```python
from build123d import *

# Parameters (mm, degrees)
SKETCH3_W           = 39.5
SKETCH3_H           = 50
SKETCH3_W_2         = 33.5
SKETCH3_H_2         = 44
BOSS_EXTRUDE1_DEPTH = 2
SKETCH4_W           = 39.5
SKETCH4_H           = 50
BOSS_EXTRUDE2_DEPTH = 1.5
SKETCH5_W           = 1.5
SKETCH5_H           = 11
CUT_EXTRUDE1_DEPTH  = 3
SKETCH7_W           = 39.5
SKETCH7_H           = 50
SKETCH7_W_2         = 28.5
SKETCH7_H_2         = 30.1
BOSS_EXTRUDE3_DEPTH = 1
SKETCH8_W           = 3
SKETCH8_H           = 6.1
SKETCH8_H_2         = 20.2
CUT_EXTRUDE2_DEPTH  = 4.5


with BuildPart() as part:
    # Sketch3 → Boss-Extrude1 (new body)
    with BuildSketch(Plane(origin=(0, 0, 0), x_dir=(1, 0, 0), z_dir=(0, 1, 0))):
        with Locations((19.75, 25)):
            Rectangle(SKETCH3_W, SKETCH3_H)
        with Locations((19.75, 25)):
            Rectangle(SKETCH3_W_2, SKETCH3_H_2, mode=Mode.SUBTRACT)
    extrude(amount=BOSS_EXTRUDE1_DEPTH)

    # Sketch4 → Boss-Extrude2 (add)
    with BuildSketch(Plane(origin=(0, 2, 0), x_dir=(1, 0, 0), z_dir=(0, 1, 0))):
        with Locations((19.75, 25)):
            Rectangle(SKETCH4_W, SKETCH4_H)
    extrude(amount=BOSS_EXTRUDE2_DEPTH)

    # Sketch5 → Cut-Extrude1 (cut)
    with BuildSketch(Plane(origin=(0, 3.5, 0), x_dir=(1, 0, 0), z_dir=(0, 1, 0))):
        with Locations((4.956023136, 23.5)):
            Rectangle(SKETCH5_W, SKETCH5_H)
    extrude(amount=-CUT_EXTRUDE1_DEPTH, mode=Mode.SUBTRACT)

    # Sketch7 → Boss-Extrude3 (add)
    with BuildSketch(Plane(origin=(0, 3.5, 0), x_dir=(1, 0, 0), z_dir=(0, 1, 0))):
        with Locations((19.75, 25)):
            Rectangle(SKETCH7_W, SKETCH7_H)
        with Locations((18.45, 23.55)):
            Rectangle(SKETCH7_W_2, SKETCH7_H_2, mode=Mode.SUBTRACT)
    extrude(amount=BOSS_EXTRUDE3_DEPTH)

    # Sketch8 → Cut-Extrude2 (cut)
    with BuildSketch(Plane.XZ):
        with Locations((1.5, -3.05)):
            Rectangle(SKETCH8_W, SKETCH8_H)
        with Locations((1.5, -25)):
            Rectangle(SKETCH8_W, SKETCH8_H_2)
        with Locations((1.5, -46.95)):
            Rectangle(SKETCH8_W, SKETCH8_H)
        with Locations((38, -3.05)):
            Rectangle(SKETCH8_W, SKETCH8_H)
        with Locations((38, -25)):
            Rectangle(SKETCH8_W, SKETCH8_H_2)
        with Locations((38, -46.95)):
            Rectangle(SKETCH8_W, SKETCH8_H)
    extrude(amount=-CUT_EXTRUDE2_DEPTH, mode=Mode.SUBTRACT)


solid = part.part
```
Design review of the part built by this model. Coordinates are the model's own, in mm. A direction names the side the tool comes from. Give positions to 0.01 mm unless a question says otherwise; leave off trailing zeros. Order: outer loops, then holes, each group sorted by start corner. A loop starts at its lowest first (then second) coordinate and runs counter-clockwise, first axis right, second up. Notation, with made-up numbers: M 89.5,-35 L 120.5,-35 A16 ccw 120.5,-6 Z; hole C -11.75,31 d7. An arc over 180 degrees is marked long. One line per question, with ' | ' between items. Start each with the question number.
Q1. We need section B-B (y = 0.6). Write out the cut boundary in (x, z), plus the area to 3 significant figures.
Q2. For L1, parallel to Z at x = 30, y = 1.1; L2, parallel to Z at x = 31, y = 4.15; L3, parallel to X at y = 1.8, z = -8, list the stretches that pass through material, from the lowest coordinate up. Write a range as [from, to].
Q3. We need section C-C (z = -17). Write out the cut boundary in (x, y), plus the area to 4 significant figures.
Q4. For pin 1 Ø0.5 at (y, z) = (4, -30) entering from -X; pin 2 Ø1.1 at (y, z) = (4, -18.5) entering from +X; pin 3 Ø1 at (x, z) = (4.5, -35) entering from -Y, all flat-tipped, find the tip position at first contact; note any pin that passes through.
Q5. The part is to be moulded in two halves that separate along Z. For faces 1 (the face through (1, 2, -6.1)), 2 (the face through (20, 0, -49)), 3 (the face through (32.7, 4, -23)), say which applies: +Z half, -Z half, draft (parallel to the pull), parting line (faces both ways), or undercut.
Q6. Machinability: for faces 4 (the face through (36.5, 3, -48)), 5 (the face through (4.206, 3, -23)), 6 (the face through (1, 2, -14.9)), which of the approach directions +Z, -Z, +X, -X, +Y, -Y give a long, thin tool a straight path to every point of the face, cutting with its end or side? Answer none if there is none.
Q7. We need section D-D (x = 14). Write out the cut boundary in (y, z).
Returned:
1) outline: M 0,-43.9 L 3,-43.9 L 3,-35.1 L 0,-35.1 Z; M 0,-14.9 L 3,-14.9 L 3,-6.1 L 0,-6.1 Z; M 3,-50 L 36.5,-50 L 36.5,-47 L 3,-47 Z; M 3,-3 L 36.5,-3 L 36.5,0 L 3,0 Z; M 36.5,-43.9 L 39.5,-43.9 L 39.5,-35.1 L 36.5,-35.1 Z; M 36.5,-14.9 L 39.5,-14.9 L 39.5,-6.1 L 36.5,-6.1 Z | area: 307 mm2
2) L1: [-50, -47], [-3, 0] | L2: [-50, -38.6], [-8.5, 0] | L3: [0, 3], [36.5, 39.5]
3) outline: M 3,2 L 36.5,2 L 36.5,4.5 L 32.7,4.5 L 32.7,3.5 L 4.2,3.5 L 4.2,4.5 L 3,4.5 Z | area: 55.25 mm2
4) pin 1: x = 3 | pin 2: x = 36.5 | pin 3: y = 2
5) face 1: +Z half | face 2: draft | face 3: undercut
6) face 4: -Z, +X, +Y, -Y | face 5: +Y, -Y | face 6: -X, +Y, -Y
7) outline: M 0,-50 L 4.5,-50 L 4.5,-38.6 L 3.5,-38.6 L 3.5,-8.5 L 4.5,-8.5 L 4.5,0 L 0,0 L 0,-3 L 2,-3 L 2,-47 L 0,-47 Z
